Input: dimensioned drawing with shaded views. Units: mm. Origin: part minimum x, y, z. Round coordinates to 2 decimals unless told otherwise and drop trailing zeros. Write each loop counter-clockwise with the first axis right and the second up, starting at its lowest first coordinate (ties: lowest second). Pieces come first, ordered by that corner, then holes. Notation, with made-up numbers: (-18.5, 11) - (7.5, 11) arc R14 ccw to (7.5, 21) - close; hole circle Ø10 at (85, 6). An arc over 180 degrees is marked (long way). Use one line per item in the form item = value.
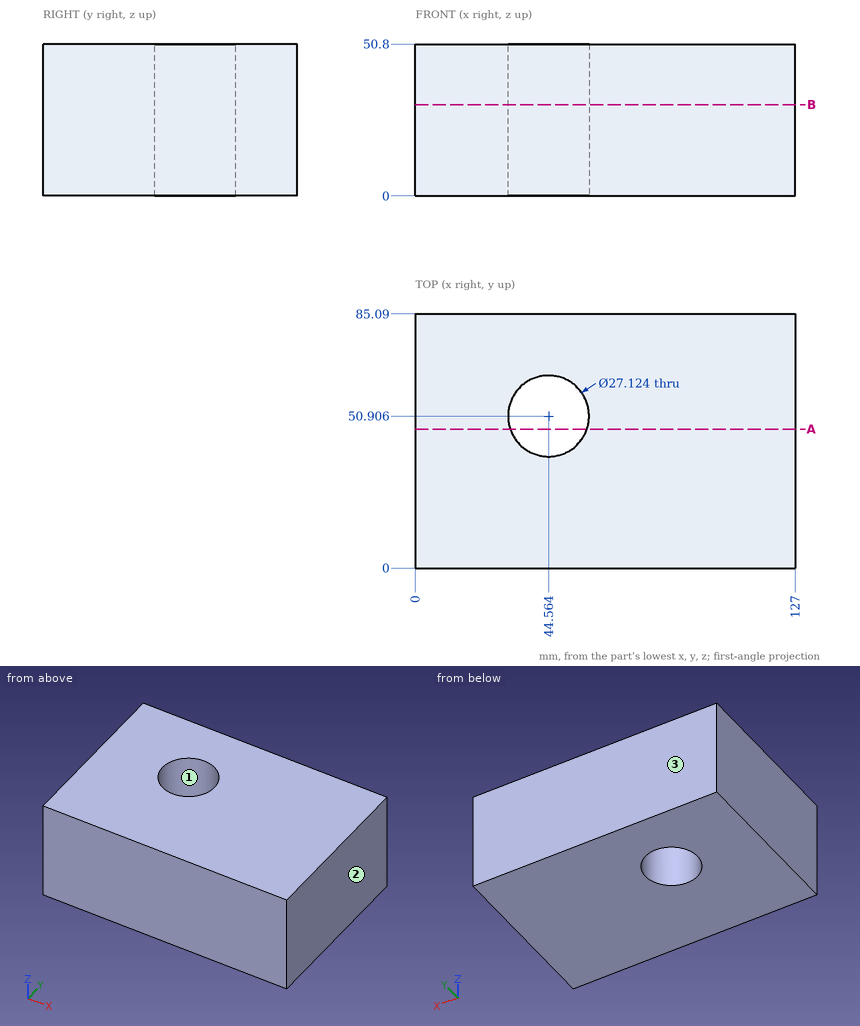
(1) Draft query along X for the marked faces 1, 2 and 3. Return one class per face: released by +X, released by -X, zero draft, split by the parting line, or undercut.
Derived:
face_1 = undercut
face_2 = released by +X
face_3 = zero draft
(2) Cut plane A-A on y = 46.5. Output: boundary loops of the cut face in (x, z).
Derived:
outline = (0, 0) - (31.74, 0) - (31.74, 50.8) - (0, 50.8) - close; (57.39, 0) - (127, 0) - (127, 50.8) - (57.39, 50.8) - close
(3) Material intervals for L1, parallel to Y at x = 45, z = 23; L2, parallel to X at y = 56.5, z = 3; L3, parallel to X at y = 61.5, z = 36.5 (1 decimal), sorted ascending.
Derived:
L1 = 0 to 37.35, 64.46 to 85.09
L2 = 0 to 32.21, 56.92 to 127
L3 = 0 to 36.1, 53 to 127
(4) Cut plane B-B on z = 30.5. Output: boundary loops of the cut face in (x, y) (1 decimal).
Derived:
outline = (0, 0) - (127, 0) - (127, 85.1) - (0, 85.1) - close; hole circle Ø27.1 at (44.6, 50.9)
